```python
from build123d import *

# Parameters (mm, degrees)
SKETCH5_R           = 30
SKETCH5_R_2         = 7
BOSS_EXTRUDE5_DEPTH = 25
SKETCH5_6_R         = 7
BOSS_EXTRUDE6_DEPTH = 25
SKETCH5_8_R         = 3.5
CUT_EXTRUDE1_DEPTH  = 25
BOSS_EXTRUDE7_START = -25
SKETCH5_9_R         = 7
SKETCH5_9_R_2       = 3.5
BOSS_EXTRUDE7_DEPTH = 25


with BuildPart() as part:
    # Sketch5 → Boss-Extrude5 (new body)
    with BuildSketch(Plane(origin=(0, 0, 0), x_dir=(1, 0, 0), z_dir=(0, 1, 0))):
        with Locations(Location((0, 0, 0), (0, 0, 270))):
            Circle(SKETCH5_R)
        with Locations(Location((0, 0, 0), (0, 0, 270))):
            Circle(SKETCH5_R_2, mode=Mode.SUBTRACT)
    extrude(amount=BOSS_EXTRUDE5_DEPTH)

    # Sketch5_6 → Boss-Extrude6 (add)
    with BuildSketch(Plane(origin=(0, 0, 0), x_dir=(1, 0, 0), z_dir=(0, 1, 0))):
        Circle(SKETCH5_6_R)
    extrude(amount=BOSS_EXTRUDE6_DEPTH)

    # Sketch5_8 → Cut-Extrude1 (cut)
    with BuildSketch(Plane(origin=(0, 0, 0), x_dir=(1, 0, 0), z_dir=(0, 1, 0))):
        with Locations(Location((0, 0, 0), (0, 0, 270))):
            Circle(SKETCH5_8_R)
    extrude(amount=CUT_EXTRUDE1_DEPTH, mode=Mode.SUBTRACT)

    # Sketch5_9 → Boss-Extrude7 (add)
    with BuildSketch(Plane(origin=(0, 0, 0), x_dir=(1, 0, 0), z_dir=(0, 1, 0)).offset(BOSS_EXTRUDE7_START)):
        with Locations(Location((0, 0, 0), (0, 0, 270))):
            Circle(SKETCH5_9_R)
        with Locations(Location((0, 0, 0), (0, 0, 270))):
            Circle(SKETCH5_9_R_2, mode=Mode.SUBTRACT)
    extrude(amount=BOSS_EXTRUDE7_DEPTH)

    # Sketch9 → CBORE for M5 Hex Head Bolt1 (revolve, cut)
    with BuildSketch(Plane(origin=(0, -10.718846388, 10), x_dir=(0, -1, 0), z_dir=(1, 0, 0))):
        Polygon((0, 0), (0, 40), (2.75, 40), (2.75, 3.58), (6.12, 3.58), (6.12, 0.025), (6.145, 0), align=None)
    revolve(axis=Axis((0, -10.718846388, 16.35), (0, 0, -1)), mode=Mode.SUBTRACT)


solid = part.part
```
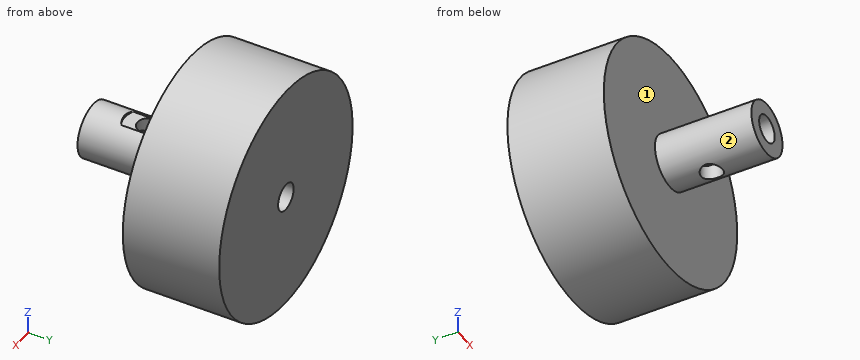
Build history of the part. All positions in model axes, mm. Face numbers are marked on the shaded views. Coordinates: 2 decimals unless noted, no trailing zeros. Order: outer loops, then holes, each group sorted by start corner. A loop starts at its lowest first (then second) coordinate and runs counter-clockwise, first axis right, second up. Notation, with made-up numbers: (74, 27) -> (95, 27) arc R20 ccw to (95, 50) -> close; hole circle Ø9 at (19, -26.5). An arc over 180 degrees is marked (long way). Answer in a Markdown table with one row per item. Add a question column.
Q1. Drop flat-ended pins along their axis: pin 1 (8 mm diameter, centred on y = 16, z = -9, fed in from -X); pin 2 (4 mm diameter, centred on x = 11.5, z = 3, fed in from -Y); pin 3 (3 mm diameter, centred on y = 17.5, z = 12.5, fed in from -X); pin 4 (6.5 mm diameter, centred on x = 0, z = 0, fed in from -Y). Give the stop position or say it passes through.
Q2. Band-saw the part on A-A, the plane x = 0. List the corners of the cut face in (y, z), then the cut area to 3 significant figures.
Q3. Band-saw the part on B-B, the plane z = 0. List the corners of the cut face in (x, y), then the cut area to 3 significant figures.
Q4. Band-saw the part on D-D, the plane x = 19. List the corners of the cut face in (y, z), then the cut area to 3 significant figures.
Q5. Band-saw the part on C-C, the plane y = 7.5. List the corners of the cut face in (x, z), then the cut area to 3 significant figures.
Q6. Wall check: line 1 along X through (y, z) = (4, 0); line 2 along Z through (x, y) = (-2, -14); line 3 along Y through (x, z) = (3.5, 18.5). Give the ranges that are in metal, low to high. Write a range as [from, to].
Q7. Mould opens along Z. For the marked faces 1 and 2 say: +Z half, -Z half, draft (parallel to the pull), parting line (faces both ways), or undercut.
Answers follow:
| question | item | result |
|---|---|---|
| 1 | pin 1 | x = -29.58 |
| 1 | pin 2 | y = 0 |
| 1 | pin 3 | x = -27.91 |
| 1 | pin 4 | through |
| 2 | outline | (-25, -7) -> (-13.47, -7) -> (-13.47, -3.5) -> (-25, -3.5) -> close; (-25, 3.5) -> (-13.47, 3.5) -> (-13.47, 6.42) -> (-16.84, 6.42) -> (-16.84, 7) -> (-25, 7) -> close; (-7.97, -7) -> (0, -7) -> (0, -30) -> (25, -30) -> (25, -3.5) -> (-7.97, -3.5) -> close; (-7.97, 3.5) -> (25, 3.5) -> (25, 30) -> (0, 30) -> (0, 7) -> (-4.6, 7) -> (-4.6, 6.42) -> (-7.97, 6.42) -> close |
| 2 | area | 1,460 mm^2 |
| 3 | outline | (-30, 0) -> (-7, 0) -> (-7, -25) -> (-3.5, -25) -> (-3.5, 25) -> (-30, 25) -> close; (3.5, -25) -> (7, -25) -> (7, 0) -> (30, 0) -> (30, 25) -> (3.5, 25) -> close |
| 3 | area | 1,500 mm^2 |
| 4 | outline | (0, -23.22) -> (25, -23.22) -> (25, 23.22) -> (0, 23.22) -> close |
| 4 | area | 1,160 mm^2 |
| 5 | outline | circle Ø60 at (0, 0); hole circle Ø7 at (0, 0) |
| 5 | area | 2,790 mm^2 |
| 6 | line 1 | [-30, -3.5], [3.5, 30] |
| 6 | line 2 | [-6.71, -2.87], [2.87, 6.42] |
| 6 | line 3 | [0, 25] |
| 7 | face 1 | draft |
| 7 | face 2 | parting line |
